from build123d import *

# Parameters (mm, degrees)
SKETCH2_R           = 9.525
SKETCH2_R_2         = 6
BOSS_EXTRUDE1_DEPTH = 60
CUT_EXTRUDE1_START  = 2.5
SKETCH5_W           = 4
SKETCH5_H           = 4
CUT_EXTRUDE1_DEPTH  = 25


with BuildPart() as part:
    # Sketch1 → Revolve1 (revolve)
    with BuildSketch(Plane(origin=(0, 0, 0), x_dir=(0, 0, -1), z_dir=(1, 0, 0))):
        Polygon((0, 6), (0, 25), (-3, 25), (-3, 0), (27.090074414, 0), (28, 2.5), (40, 2.5), (40, 6), align=None)
    revolve(axis=Axis((0, 0, -27.090074414), (0, 0, 1)))

    # Sketch2 → Boss-Extrude1 (add)
    with BuildSketch(Plane.XY.offset(3)):
        with Locations((0, -8.4375)):
            Circle(SKETCH2_R)
        with Locations((0, -8.4375)):
            Circle(SKETCH2_R_2, mode=Mode.SUBTRACT)
    extrude(amount=BOSS_EXTRUDE1_DEPTH)

    # Sketch5 → Cut-Extrude1 (cut)
    with BuildSketch(Plane(origin=(0, 0, 0), x_dir=(-1, 0, 0), z_dir=(0, 0, -1)).offset(CUT_EXTRUDE1_START)):
        with Locations((0, -5.8)):
            Rectangle(SKETCH5_W, SKETCH5_H)
    cut_extrude1 = extrude(amount=CUT_EXTRUDE1_DEPTH, mode=Mode.SUBTRACT)

    # Mirror1: Cut-Extrude1 across plane
    add(cut_extrude1.mirror(Plane.ZX), mode=Mode.SUBTRACT)


solid = part.part
Design review of the part built by this model. Coordinates are the model's own, in mm. A direction names the side the tool comes from. Coordinates: 2 decimals unless noted, no trailing zeros. Order: outer loops, then holes, each group sorted by start corner. A loop starts at its lowest first (then second) coordinate and runs counter-clockwise, first axis right, second up. Notation, with made-up numbers: (-4, 89.25) -> (36, 89.25) arc R26 ccw to (36, 109.25) -> close; hole circle Ø7 at (60, 12.5). An arc over 180 degrees is marked (long way). Use one line per item in the form item = value. Start each with the question number.
(1) Insertion check: pin 1 (7 mm diameter, centred on x = 0, y = -8.44, fed in from +Z); pin 2 (1 mm diameter, centred on x = 6, z = 40, fed in from +Y); pin 3 (0.9 mm diameter, centred on y = -5, z = -15.5, fed in from -X); pin 4 (6 mm diameter, centred on x = -17.5, z = -5, fed in from -Y). Each pin has a flat end and moves straight along its axis. Give the tip position at first contact, or say it passes through.
(2) Add section C-C on y = 14.5. State the section outline as (x, z) points, plus the area to 3 significant figures.
(3) For probe 1 along Y at (x, z) = (0, 45.5); probe 2 along Y at (x, z) = (0, -35), list the stretches that pass through material, from the lowest coordinate up.
(4) Add section A-A on z = -13.5. State the section outline as (x, y) points.
(5) Add section D-D on x = -11. State the section outline as (y, z) points, plus the area to 3 significant figures.
(6) For faces 1 (the flat face through (6.2, -8.3, 63)), 2 (the cylindrical face through (5.857, -1.301, -19.72)), 3 (the flat face through (0, -5, -27.5)), 4 (the flat face through (0, 3.8, -15)), 5 (the flat face through (0, -9, 3)), list the 3-axis set-ups (+Z, -Z, +X, -X, +Y, -Y) from which the entire face can be reached by the end or side of a thin tool; tool diameter is ignored.
(7) The part is to be moulded in two halves that separate along Y. For faces 6 (the cylindrical face through (-2.065, -17.736, 32.58)), 7 (the flat face through (0, -3, -40)), 8 (the cylindrical face through (2.44, -0.54, -34.08)), say which applies: +Y half, -Y half, draft (parallel to the pull), parting line (faces both ways), or undercut.
(8) Add section B-B on z = -33. State the section outline as (x, y) points.
Answer block:
q1.pin_1 = 3
q1.pin_2 = -0.66
q1.pin_3 = -3.91
q1.pin_4 = through
q2.outline = (-20.37, 0) -> (20.37, 0) -> (20.37, 3) -> (-20.37, 3) -> close
q2.area = 122 mm²
q3.probe_1 = -17.96 to -14.44, -2.44 to 1.09
q3.probe_2 = -6 to -2.5, 2.5 to 6
q4.outline = (-2, -5.66) -> (-2, -3.8) -> (2, -3.8) -> (2, -5.66) arc R6 ccw to (2, 5.66) -> (2, 3.8) -> (-2, 3.8) -> (-2, 5.66) arc R6 ccw to start
q5.outline = (-22.45, 0) -> (22.45, 0) -> (22.45, 3) -> (-22.45, 3) -> close
q5.area = 135 mm²
q6.face_1 = +Z, +X, -X, +Y, -Y
q6.face_2 = -Z
q6.face_3 = -Y
q6.face_4 = +Y
q6.face_5 = +Z
q7.face_6 = parting line
q7.face_7 = draft
q7.face_8 = undercut
q8.outline = circle Ø12 at (0, 0); hole circle Ø5 at (0, 0)
